Design review of the part shown in the three views and the two pictorial views. Dimensions are in mm from the part's minimum x, y and z. A direction names the side the tool comes from. Round coordinates to 2 decimals unless told otherwise and drop trailing zeros. Write each loop counter-clockwise with the first axis right and the second up, starting at its lowest first coordinate (ties: lowest second). Pieces come first, ordered by that corner, then holes. Notation, with made-up numbers: (15.5, -23.75) - (57.5, -23.75) arc R32 cw to (57.5, 10.25) - close; hole circle Ø2 at (81, 49). An arc over 180 degrees is marked (long way). Use one line per item in the form item = value.
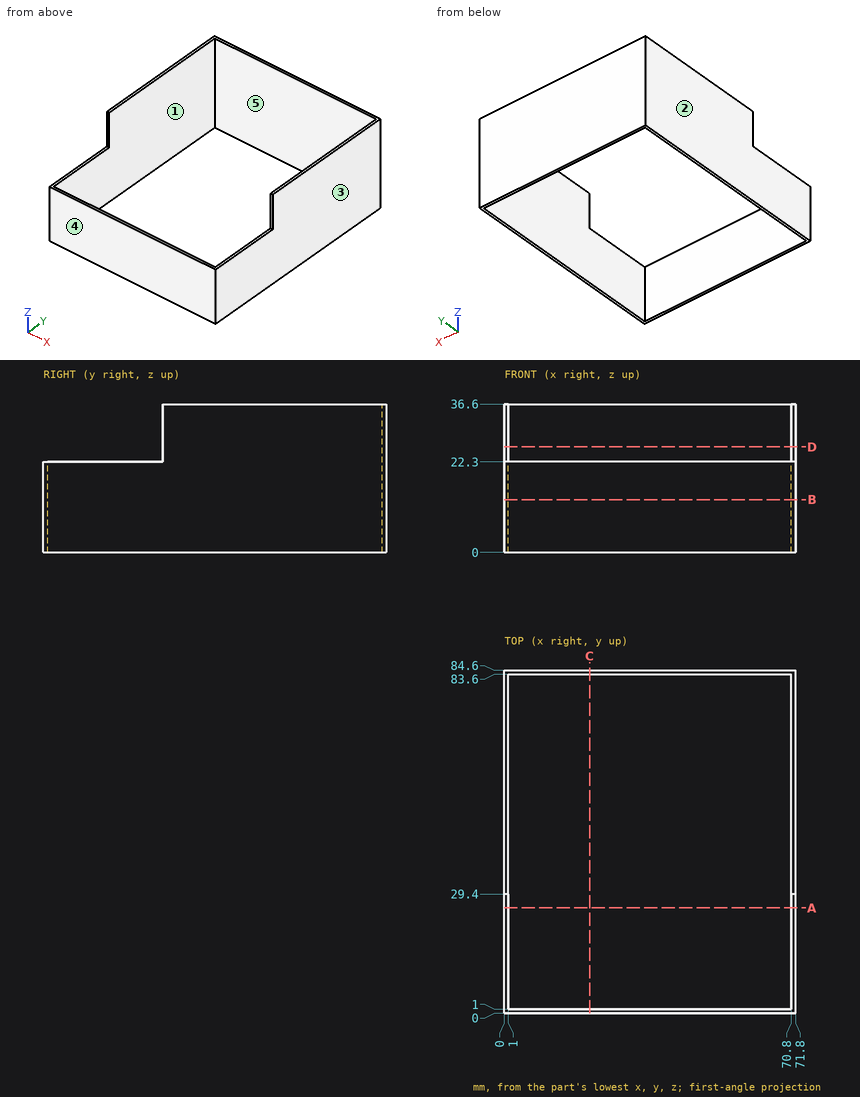
Q1. We need section A-A on y = 26. Write out the cut boundary in (x, z).
Calculated:
outline = (0, 0) - (1, 0) - (1, 22.3) - (0, 22.3) - close; (70.8, 0) - (71.8, 0) - (71.8, 22.3) - (70.8, 22.3) - close
Q2. We need section D-D on z = 26. Write out the cut boundary in (x, y), then the cut area to 3 significant figures.
Calculated:
outline = (0, 29.4) - (1, 29.4) - (1, 83.6) - (70.8, 83.6) - (70.8, 29.4) - (71.8, 29.4) - (71.8, 84.6) - (0, 84.6) - close
area = 180 mm2
Q3. For P1, Ø0.5, axis at x = 71.5, z = 33, coming from the -Y side, flat-tipped, find the tip position at first contact; note if it passes through.
Calculated:
P1 = 29.4
Q4. We need section B-B on z = 13. Write out the cut boundary in (x, y).
Calculated:
outline = (0, 0) - (71.8, 0) - (71.8, 84.6) - (0, 84.6) - close; hole (1, 1) - (70.8, 1) - (70.8, 83.6) - (1, 83.6) - close
Q5. We need section C-C on x = 21. Write out the cut boundary in (y, z).
Calculated:
outline = (0, 0) - (1, 0) - (1, 22.3) - (0, 22.3) - close; (83.6, 0) - (84.6, 0) - (84.6, 36.6) - (83.6, 36.6) - close
Q6. Draft analysis for pull direction X (two halves, no side actions). For the marked faces 1, 2 and 3, state which applies: released by +X, released by -X, zero draft, split by the parting line, or undercut.
Calculated:
face_1 = undercut
face_2 = released by -X
face_3 = released by +X
Q7. To check wall thickness, follow line 1 along X through (y, z) = (79, 13); line 2 along Y through (x, z) = (35.5, 18); line 3 along Y through (x, z) = (11, 29). State the ranges of each line that lie inside material, in increasing order. Write a range as from..to.
Calculated:
line_1 = 0..1, 70.8..71.8
line_2 = 0..1, 83.6..84.6
line_3 = 83.6..84.6
Q8. Machinability: for the marked faces 4 and 5, which of the approach directions +Z, -Z, +X, -X, +Y, -Y give a long, thin tool a straight path to every point of the face, cutting with its end or side? Answer none if there is none.
Calculated:
face_4 = +Z, -Z, +X, -X, -Y
face_5 = +Z, -Z
